Geometry check sheet. Reference: the model listing, model coordinates, mm. Face numbers are marked on the shaded views. A direction names the side the tool comes from. Coordinates: 2 decimals unless noted, no trailing zeros. Write each loop counter-clockwise with the first axis right and the second up, starting at its lowest first coordinate (ties: lowest second). Pieces come first, ordered by that corner, then holes. Notation, with made-up numbers: (21, 87) -> (60, 87) arc R21 cw to (60, 102) -> close; hole circle Ø5 at (61.25, -35). An arc over 180 degrees is marked (long way). Answer in a Markdown table with one row per item. Add a question column.
Q1. Section check A-A, the plane y = 226. Record the boundary of the cut face in (x, z).
Q2. Section check B-B, the plane z = 11.5. Record the boundary of the cut face in (x, y), and give its area (3 significant figures).
Q3. Thickness scan on line 1 (Y direction, x = 25, z = 37.3); line 2 (X direction, y = -300, z = 38.15); line 3 (Z direction, x = 13, y = 230.5). Record the ranges inside material, lowest first.
Q4. Gauge pin test, flat ends, axial feed: P1, Ø18, axis at y = 160, z = 13, coming from the +X side; P2, Ø11, axis at x = 27.5, y = -153, coming from the -Z side. Record the tip position at first contact, or that the pin passes through.
Q5. Tool access check on the marked faces 1 and 2. Record the directions out of +Z, -Z, +X, -X, +Y, -Y that give a thin tool (end or side, any length) a straight path to the whole face; none if there is none.
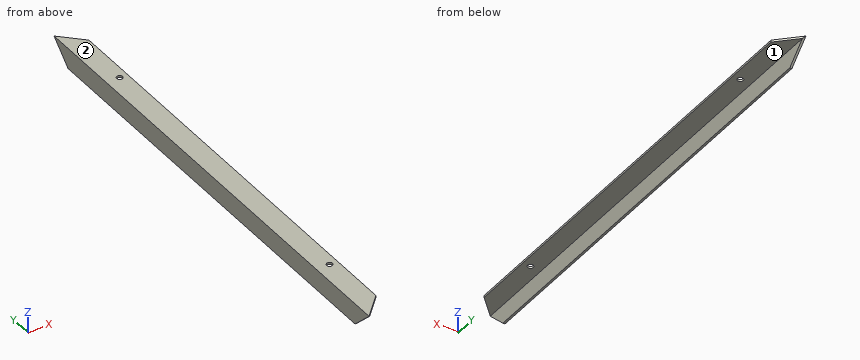
```python
from build123d import *

# Parameters (mm, degrees)
F1_DEPTH = 450
F3_DEPTH = 40
F5_DEPTH = 40
F7_D     = 11


with BuildPart() as f1:
    # F0 (on Front) → F1 (new body, symmetric)
    with BuildSketch(Plane.XZ):
        Polygon((0, 40), (0, 0), (4, 0), (4, 36), (40, 36), (40, 40), align=None)
    extrude(amount=F1_DEPTH, both=True)

    # F2 (on face) → F3 (cut)
    with BuildSketch(Plane(origin=(0, 0, 0), x_dir=(0, -1, 0), z_dir=(-1, 0, 0))):
        Polygon((-410, 0), (-450, 40), (-450, 0), align=None)
        Polygon((450, 0), (450, 40), (410, 0), align=None)
    extrude(amount=-F3_DEPTH, mode=Mode.SUBTRACT)

    # F4 (on face) → F5 (cut)
    with BuildSketch(Plane.XY.offset(40)):
        Polygon((40, 450), (0, 450), (40, 410), align=None)
        Polygon((40, -410), (0, -450), (40, -450), align=None)
    extrude(amount=-F5_DEPTH, mode=Mode.SUBTRACT)

    # F7 (through all)
    with Locations(Plane.XY.offset(40)):
        with Locations((25, -300), (25, 300)):
            Hole(F7_D / 2)


solid = f1.part
```
Calculated:
| question | item | result |
|---|---|---|
| 1 | outline | (0, 0) -> (4, 0) -> (4, 36) -> (40, 36) -> (40, 40) -> (0, 40) -> close |
| 2 | outline | (0, -421.5) -> (4, -421.5) -> (4, 421.5) -> (0, 421.5) -> close |
| 2 | area | 3,370 mm² |
| 3 | line 1 | y = -425 to -305.5, -294.5 to 294.5, 305.5 to 425 |
| 3 | line 2 | x = 0 to 19.5, 30.5 to 40 |
| 3 | line 3 | z = 36 to 40 |
| 4 | P1 | stops at x = 4 |
| 4 | P2 | stops at z = 36 |
| 5 | face 1 | -Z, +X, +Y, -Y |
| 5 | face 2 | +Z, +X, -X, +Y, -Y |
